For this review, use the dimensioned drawing (mm, ordinates from the lowest corner) and the shaded views. A direction names the side the tool comes from. Coordinates: 2 decimals unless noted, no trailing zeros. Write each loop counter-clockwise with the first axis right and the second up, starting at its lowest first coordinate (ties: lowest second). Pieces come first, ordered by that corner, then holes. Notation, with made-up numbers: M -25,27 L -17,27 A13 cw -17,49 Z; hole C 67,19.5 d2. An arc over 180 degrees is marked long. One line per question, with ' | ' between items.
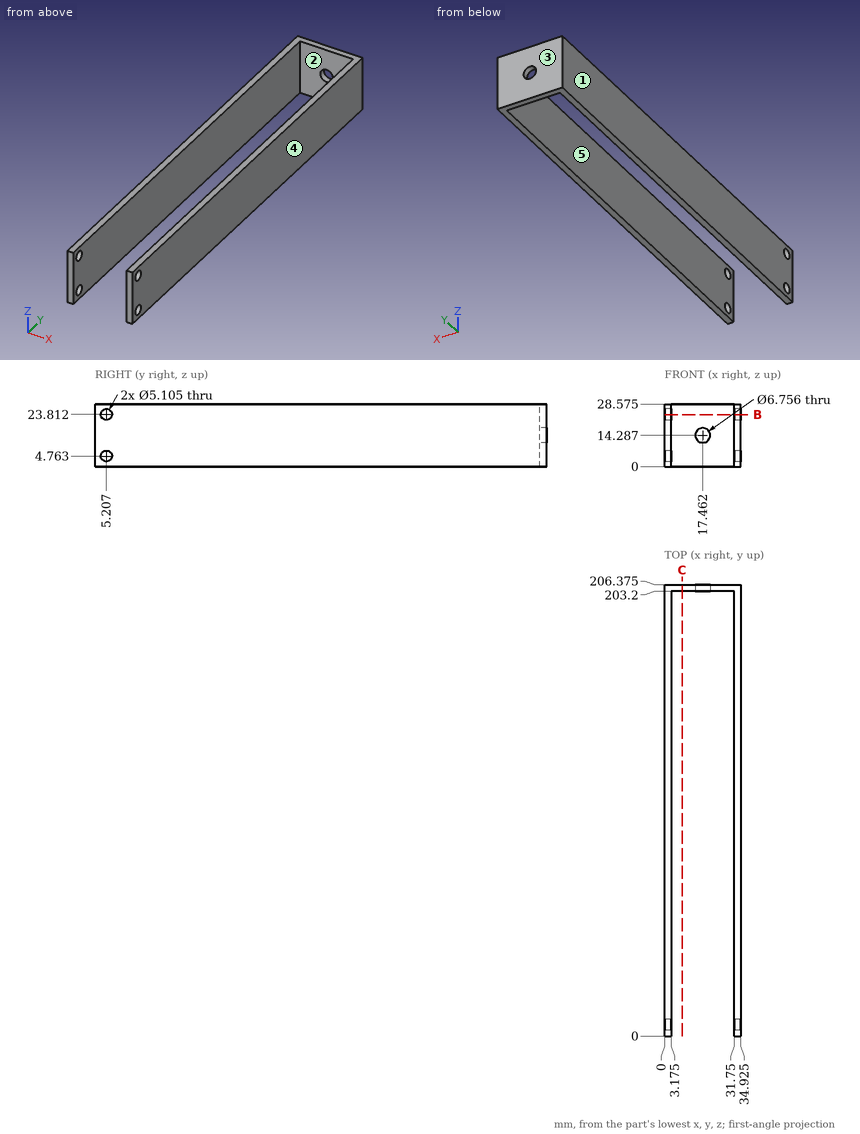
1. Draft analysis for pull direction X (two halves, no side actions). For the marked faces 1, 2 and 3, state which applies: pulls with the +X half, pulls with the -X half, needs draft (parallel to the pull), parting line crosses it, or undercut.
Answer sheet:
face 1: pulls with the -X half | face 2: undercut | face 3: needs draft
2. Take a section at B-B (z = 23.75). Count the separate pieces of the cut face and the enclosed holes in it, then the cut area to 3 significant figures.
Answer sheet:
separate pieces: 3 | enclosed holes: 0 | area: 1,370 mm^2
3. Tool access review of the marked faces 4 and 5: name each direction out of +Z, -Z, +X, -X, +Y, -Y from which nothing blocks a thin tool from reaching the whole face with its end or side.
Answer sheet:
face 4: +Z, -Z, +X, +Y, -Y | face 5: +Z, -Z, -Y
4. Take a section at C-C (x = 8). Write out the cut boundary in (y, z) (1 decimal).
Answer sheet:
outline: M 203.2,0 L 206.4,0 L 206.4,28.6 L 203.2,28.6 Z
5. To check wall thickness, follow line 1 along Y through (x, z) = (29, 5.75) (1 decimal); line 2 along Y through (x, z) = (33.5, 4.25) (1 decimal). State the ranges of each line that lie inside material, in increasing order. Write a range as [from, to].
Answer sheet:
line 1: [203.2, 206.4] | line 2: [0, 2.7], [7.7, 206.4]
6. Insertion check: pin 1 Ø12 at (x, z) = (17.5, 4.5) entering from -Y. The pin has a flat end and moves straight along its axis. Give the tip position at first contact, or say it passes through.
Answer sheet:
pin 1: y = 203.2
